Design review of the part built by this model. Coordinates are the model's own, in mm. Face numbers are marked on the shaded views. A direction names the side the tool comes from. Give positions to 0.01 mm unless a question says otherwise; leave off trailing zeros. Loops run counter-clockwise (first coordinate to the right, second up) from the corner with the lowest first, then second, coordinate; pieces in that order, holes last. Notation, with made-up numbers: (0, 21.25) -> (55, 21.25) arc R18 cw to (55, 36.25) -> close; hole circle Ø5 at (53, -32.5). An arc over 180 degrees is marked (long way). Use a Markdown table: item, result. Add a question column.
1. Add section D-D (y = 3.5). State the section outline as (x, z) points, and give its area (3 significant figures).
2. To check wall thickness, follow line 1 (Y direction, x = 3.5, z = -1.2); line 2 (Z direction, x = -1, y = 3); line 3 (X direction, y = 2, z = 0.45). State the ranges of each line that lie inside material, in increasing order.
3. For the marked faces 1, 2, 3 and 4, list the 3-axis set-ups (+Z, -Z, +X, -X, +Y, -Y) from which the entire face can be reached by the end or side of a thin tool; tool diameter is ignored.
4. Add section B-B (x = -1). State the section outline as (y, z) points.
5. Add section C-C (z = -1.15). State the section outline as (x, y) points, and give its area (3 significant figures).
6. Add section A-A (y = -6). State the section outline as (x, z) points, and give its area (3 significant figures).
7. For pin 1 Ø2 at (x, y) = (-1, -2) entering from -Z; pin 2 Ø1.2 at (x, z) = (-1.5, 0.5) entering from -Y; pin 3 Ø0.8 at (y, z) = (4, -0.5) entering from +X; pin 4 Ø1.2 at (x, y) = (-0.5, 3.5) entering from -Z, all flat-tipped, find the tip position at first contact; note any pin that passes through.
```python
from build123d import *

# Parameters (mm, degrees)
SKETCH1_W           = 8.5
SKETCH1_H           = 3.8
BOSS_EXTRUDE1_DEPTH = 2
SKETCH2_W           = 1.5
SKETCH2_H           = 1.5
BOSS_EXTRUDE2_DEPTH = 3
SKETCH3_W           = 0.125
SKETCH3_H           = 0.125
BOSS_EXTRUDE3_DEPTH = 5


with BuildPart() as part:
    # Sketch1 → Boss-Extrude1 (new, symmetric)
    with BuildSketch(Plane.XY):
        Rectangle(SKETCH1_W, SKETCH1_H)
    extrude(amount=BOSS_EXTRUDE1_DEPTH, both=True)

    # Sketch2 → Boss-Extrude2 (add)
    with BuildSketch(Plane(origin=(0, 1.9, 0), x_dir=(1, 0, 0), z_dir=(0, 1, 0))):
        with Locations((-1, 0)):
            Rectangle(SKETCH2_W, SKETCH2_H)
    extrude(amount=BOSS_EXTRUDE2_DEPTH)

    # Sketch3 → Boss-Extrude3 (add)
    with BuildSketch(Plane.XZ.offset(1.9)):
        Rectangle(SKETCH3_W, SKETCH3_H)
        with Locations((-2.5, 0)):
            Rectangle(SKETCH3_W, SKETCH3_H)
        with Locations((2.5, 0)):
            Rectangle(SKETCH3_W, SKETCH3_H)
    extrude(amount=BOSS_EXTRUDE3_DEPTH)


solid = part.part
```
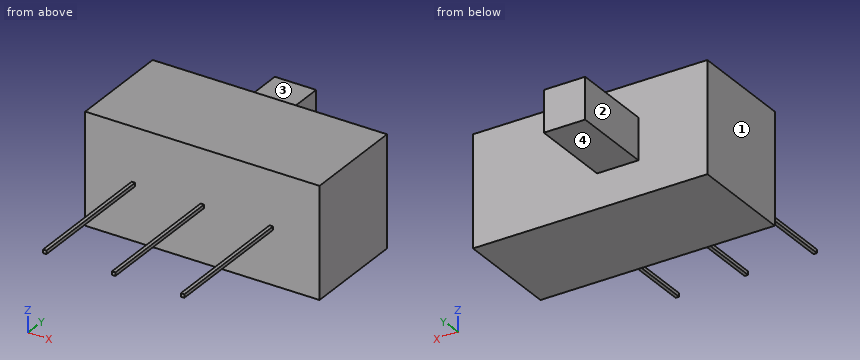
Taken from the geometry:
| question | item | result |
|---|---|---|
| 1 | outline | (-1.75, -0.75) -> (-0.25, -0.75) -> (-0.25, 0.75) -> (-1.75, 0.75) -> close |
| 1 | area | 2.25 mm^2 |
| 2 | line 1 | y = -1.9 to 1.9 |
| 2 | line 2 | z = -0.75 to 0.75 |
| 2 | line 3 | x = -1.75 to -0.25 |
| 3 | face 1 | +Z, -Z, -X, +Y, -Y |
| 3 | face 2 | +Z, -Z, -X, +Y |
| 3 | face 3 | +Z, +X, -X, +Y |
| 3 | face 4 | -Z, +X, -X, +Y |
| 4 | outline | (-1.9, -2) -> (1.9, -2) -> (1.9, -0.75) -> (4.9, -0.75) -> (4.9, 0.75) -> (1.9, 0.75) -> (1.9, 2) -> (-1.9, 2) -> close |
| 5 | outline | (-4.25, -1.9) -> (4.25, -1.9) -> (4.25, 1.9) -> (-4.25, 1.9) -> close |
| 5 | area | 32.3 mm^2 |
| 6 | outline | (-2.56, -0.06) -> (-2.44, -0.06) -> (-2.44, 0.06) -> (-2.56, 0.06) -> close; (-0.06, -0.06) -> (0.06, -0.06) -> (0.06, 0.06) -> (-0.06, 0.06) -> close; (2.44, -0.06) -> (2.56, -0.06) -> (2.56, 0.06) -> (2.44, 0.06) -> close |
| 6 | area | 0.0469 mm^2 |
| 7 | pin 1 | stops at z = -2 |
| 7 | pin 2 | stops at y = -1.9 |
| 7 | pin 3 | stops at x = -0.25 |
| 7 | pin 4 | stops at z = -0.75 |
